Source: CAD feature listing. Evaluate the final solid. Frame: model axes, mm. A direction names the side the tool comes from. Round coordinates to 2 decimals unless told otherwise and drop trailing zeros. Loops run counter-clockwise (first coordinate to the right, second up) from the corner with the lowest first, then second, coordinate; pieces in that order, holes last. Notation, with made-up numbers: M -31,-29.75 L 23,-29.75 A15 cw 23,-20.75 Z; hole C -34.5,-11 d8. An arc over 180 degrees is marked long. Answer as CSV lines item,"result". Start each with the question number.
```python
from build123d import *

# Parameters (mm, degrees)
SKICA1_W                 = 30.3
SKICA1_H                 = 5
P_IDAT_VYSUNUT_M1_DEPTH  = 5.6
SKICA2_R                 = 1.2
ODEBRAT_VYSUNUT_M1_DEPTH = 77.684092223
ODEBRAT_VYSUNUT_M3_DEPTH = 77.684092223


with BuildPart() as part:
    # Skica1 → Přidat vysunutím1 (new body)
    with BuildSketch(Plane.XY):
        Polygon((5, 0), (0, 0), (0, 65), (40.3, 65), (40.3, 0), (35.3, 0), (35.3, 60), (5, 60), align=None)
        with Locations((20.15, 32.5)):
            Rectangle(SKICA1_W, SKICA1_H)
    extrude(amount=P_IDAT_VYSUNUT_M1_DEPTH)

    # Skica2 → Odebrat vysunutím1 (cut, through all)
    with BuildSketch(Plane.ZY):
        with BuildLine():
            Line((5.6, 0), (5.6, 2.8))
            ThreePointArc((5.6, 2.8), (4.779898987, 0.820101013), (2.8, 0))
            Line((2.8, 0), (5.6, 0))
        make_face()
        with BuildLine():
            ThreePointArc((2.8, 0), (0.820101013, 0.820101013), (0, 2.8))
            Line((0, 2.8), (0, 0))
            Line((0, 0), (2.8, 0))
        make_face()
        with Locations((2.8, 2.8)):
            Circle(SKICA2_R)
    extrude(amount=-ODEBRAT_VYSUNUT_M1_DEPTH, mode=Mode.SUBTRACT)

    # Skica3 → Odebrat vysunutím3 (cut, through all)
    with BuildSketch(Plane.ZY):
        with BuildLine():
            Line((0, 65), (0, 62.2))
            ThreePointArc((0, 62.2), (0.820101013, 64.179898987), (2.8, 65))
            Line((2.8, 65), (0, 65))
        make_face()
        with BuildLine():
            ThreePointArc((2.8, 65), (4.779898987, 64.179898987), (5.6, 62.2))
            Line((5.6, 62.2), (5.6, 65))
            Line((5.6, 65), (2.8, 65))
        make_face()
    extrude(amount=-ODEBRAT_VYSUNUT_M3_DEPTH, mode=Mode.SUBTRACT)


solid = part.part
```
1) Section C-C, the plane x = 37. Return loops of the section in (y, z), and give its area (3 significant figures).
2) Contact query for flat-ended pins moving along their axis: pin 1 Ø5 at (x, y) = (32.5, 51) entering from -Z; pin 2 Ø1 at (y, z) = (50.5, 2) entering from -X; pin 3 Ø1.7 at (x, z) = (17, 3.5) entering from -Y. Output: stop coordinate, or through.
3) Section B-B, the plane y = 36. Return loops of the section in (x, z).
4) Ray query, line 1 along X through (y, z) = (22, 5); line 2 along Y through (x, z) = (1.25, 2.8); line 3 along Y through (x, z) = (28.5, 4.6). Return the intervals inside material, ascending.
5) Access query for faces 4 (the flat face through (35.3, 47, 3)), 5 (the cylindrical face through (37.76, 2.34, 3.91)), 6 (the flat face through (35.3, 15, 3)). Directions: +Z, -Z, +X, -X, +Y, -Y. A direction counts if a zero-diameter tool reaches every point of the face in a straight line with its end or side. Return the directions, or none.
6) Section A-A, the plane x = 9. Return loops of the section in (y, z).
7) Mould query, pull axis X, two halves, no side actions, for faces 1 (the flat face through (40.3, 33, 3)), 2 (the cylindrical face through (2.46, 2.34, 3.91)), 3 (the flat face through (20, 60, 3)). Classes: pulls with the +X half, pulls with the -X half, needs draft (parallel to the pull), parting line crosses it, or undercut.
Findings below:
1,outline,"M 2.8,0 L 62.2,0 A2.8 ccw 62.2,5.6 L 2.8,5.6 A2.8 ccw Z; hole C 2.8,2.8 d2.4"
1,area,"353 mm²"
2,pin 1,"through"
2,pin 2,"x = 0"
2,pin 3,"y = 30"
3,outline,"M 0,0 L 5,0 L 5,5.6 L 0,5.6 Z; M 35.3,0 L 40.3,0 L 40.3,5.6 L 35.3,5.6 Z"
4,line 1,"0 to 5, 35.3 to 40.3"
4,line 2,"0 to 1.6, 4 to 65"
4,line 3,"30 to 35, 60 to 64.34"
5,face 4,"+Z, -Z"
5,face 5,"+X, -X"
5,face 6,"+Z, -Z, -Y"
6,outline,"M 30,0 L 35,0 L 35,5.6 L 30,5.6 Z; M 60,0 L 62.2,0 A2.8 ccw 62.2,5.6 L 60,5.6 Z"
7,face 1,"pulls with the +X half"
7,face 2,"needs draft"
7,face 3,"undercut"
